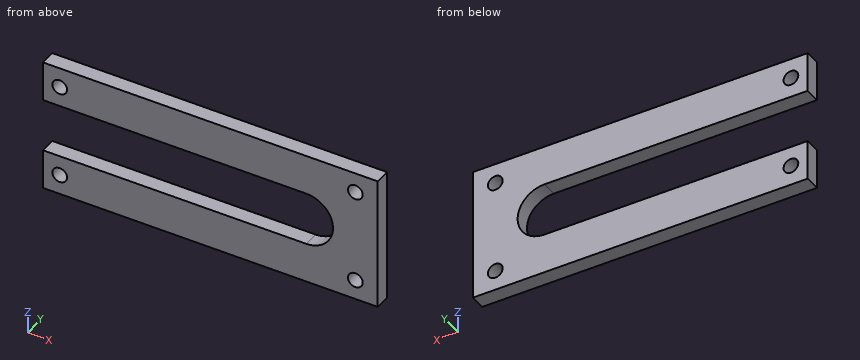
from build123d import *

# Parameters (mm, degrees)
SCHIZZO1_W                   = 150
SCHIZZO1_H                   = 7
ESTRUSIONE_ESTRUSIONE1_DEPTH = 80
SCHIZZO2_W                   = 203.570811829
SCHIZZO2_H                   = 138.674141949
SCHIZZO2_R                   = 3.3
TAGLIO_ESTRUSIONE1_DEPTH     = 171.144056611


with BuildPart() as part:
    # Schizzo1 → Estrusione-Estrusione1 (new body)
    with BuildSketch(Plane.XY):
        with Locations((75, 3.5)):
            Rectangle(SCHIZZO1_W, SCHIZZO1_H)
    extrude(amount=-ESTRUSIONE_ESTRUSIONE1_DEPTH)

    # Schizzo2 → Taglio-Estrusione1 (cut, through all)
    # profile 1 of 5: a face of its own
    with BuildSketch(Plane(origin=(0, 0, 0), x_dir=(1, 0, 0), z_dir=(0, 1, 0))):
        with Locations((73.083648688, 28.492060902)):
            Rectangle(SCHIZZO2_W, SCHIZZO2_H)
        with BuildLine():
            Line((0, 18), (118, 18))
            ThreePointArc((118, 18), (130, 30), (118, 42))
            Line((118, 42), (0, 42))
            Line((0, 42), (0, 60))
            Line((0, 60), (150, 60))
            Line((150, 60), (150, 0))
            Line((150, 0), (0, 0))
            Line((0, 0), (0, 18))
        make_face(mode=Mode.SUBTRACT)
    # profile 2 of 5: a face of its own
    with BuildSketch(Plane(origin=(0, 0, 0), x_dir=(1, 0, 0), z_dir=(0, 1, 0))):
        with Locations(Location((140, 9, 0), (0, 0, 90))):
            Circle(SCHIZZO2_R)
    # profile 3 of 5: a face of its own
    with BuildSketch(Plane(origin=(0, 0, 0), x_dir=(1, 0, 0), z_dir=(0, 1, 0))):
        with Locations(Location((140, 51, 0), (0, 0, 270))):
            Circle(SCHIZZO2_R)
    # profile 4 of 5: a face of its own
    with BuildSketch(Plane(origin=(0, 0, 0), x_dir=(1, 0, 0), z_dir=(0, 1, 0))):
        with Locations(Location((7.5, 9, 0), (0, 0, 90))):
            Circle(SCHIZZO2_R)
    # profile 5 of 5: a face of its own
    with BuildSketch(Plane(origin=(0, 0, 0), x_dir=(1, 0, 0), z_dir=(0, 1, 0))):
        with Locations(Location((7.5, 51, 0), (0, 0, 270))):
            Circle(SCHIZZO2_R)
    extrude(amount=TAGLIO_ESTRUSIONE1_DEPTH, mode=Mode.SUBTRACT)


solid = part.part
Here's how the part is built. I have some questions about the finished solid (model axes, mm). Round coordinates to 2 decimals unless told otherwise and drop trailing zeros. Loops run counter-clockwise (first coordinate to the right, second up) from the corner with the lowest first, then second, coordinate; pieces in that order, holes last. Notation, with made-up numbers: M 13.25,35 L 38.25,35 A20 ccw 38.25,72 Z; hole C 6.25,13.5 d8. An arc over 180 degrees is marked long. Write each question's results on one line, items separated by ' | '. Start each with the question number.
(1) If I drill on probe 1 along X at (y, z) = (5.25, -51); probe 2 along Z at (x, y) = (92.5, 4.5); probe 3 along X at (y, z) = (4.5, -12), over which ranges is the centre line in solid material (lowest first)? Write a range as from..to.
(2) I want a section at A-A (x = 25). Please give me the cut outline in (y, z), then the cut area to 3 significant figures.
(3) I want a section at C-C (y = 5.5). Please give me the cut outline in (x, z), then the cut area to 3 significant figures.
(4) Will this pin go through, and if not, where does the flat tip stop? P1, Ø6, axis at x = 7.5, z = -9, coming from the -Y side.
(5) I want a section at B-B (z = -9). Please give me the cut outline in (x, y), then the cut area to 3 significant figures.
(6) I want a section at D-D (x = 140). Please give me the cut outline in (y, z).
Solved:
1) probe 1: x = 0..4.2, 10.8..136.7, 143.3..150 | probe 2: z = -60..-42, -18..0 | probe 3: x = 0..6.13, 8.87..138.63, 141.37..150
2) outline: M 0,-60 L 7,-60 L 7,-42 L 0,-42 Z; M 0,-18 L 7,-18 L 7,0 L 0,0 Z | area: 252 mm²
3) outline: M 0,-60 L 150,-60 L 150,0 L 0,0 L 0,-18 L 118,-18 A12 cw 118,-42 L 0,-42 Z; hole C 7.5,-51 d6.6; hole C 7.5,-9 d6.6; hole C 140,-51 d6.6; hole C 140,-9 d6.6 | area: 5,800 mm²
4) P1: passes through
5) outline: M 0,0 L 4.2,0 L 4.2,7 L 0,7 Z; M 10.8,0 L 136.7,0 L 136.7,7 L 10.8,7 Z; M 143.3,0 L 150,0 L 150,7 L 143.3,7 Z | area: 958 mm²
6) outline: M 0,-60 L 7,-60 L 7,-54.3 L 0,-54.3 Z; M 0,-47.7 L 7,-47.7 L 7,-12.3 L 0,-12.3 Z; M 0,-5.7 L 7,-5.7 L 7,0 L 0,0 Z
